Verification items for the finished model (mm, model axes). Coordinates: 2 decimals unless noted, no trailing zeros. Order: outer loops, then holes, each group sorted by start corner. A loop starts at its lowest first (then second) coordinate and runs counter-clockwise, first axis right, second up. Notation, with made-up numbers: M 32.5,32 L 56.5,32 A32 cw 56.5,66 Z; hole C 82,27 d5. An arc over 180 degrees is marked long. Use one line per item in the form item = value. Start each with the question number.
```python
from build123d import *

# Parameters (mm, degrees)
F0_W     = 15
F0_H     = 225
F1_DEPTH = 2


with BuildPart() as f1:
    # F0 (on Front) → F1 (new body)
    with BuildSketch(Plane.XZ):
        with Locations((7.5, 112.5)):
            Rectangle(F0_W, F0_H)
        with BuildLine():
            Line((4.5, 15), (4.5, 85))
            ThreePointArc((4.5, 85), (7.5, 88), (10.5, 85))
            Line((10.5, 85), (10.5, 15))
            ThreePointArc((10.5, 15), (7.5, 12), (4.5, 15))
        make_face(mode=Mode.SUBTRACT)
        with BuildLine():
            ThreePointArc((4.5, 210), (7.5, 213), (10.5, 210))
            Line((10.5, 210), (10.5, 140))
            ThreePointArc((10.5, 140), (7.5, 137), (4.5, 140))
            Line((4.5, 140), (4.5, 210))
        make_face(mode=Mode.SUBTRACT)
    extrude(amount=F1_DEPTH)


solid = f1.part
```
1. Material ranges on line 1 along X through (y, z) = (-1.2, 186); line 2 along Z through (x, y) = (7.75, -0.6); line 3 along Z through (x, y) = (9.25, -0.6), recorded low to high.
2. Cross-section at A-A on z = 82.5. Enter the section's corners in (x, y), and give its area (3 significant figures).
3. Cross-section at B-B on x = 7.5. Enter the section's corners in (y, z), and give its area (3 significant figures).
4. Cross-section at C-C on y = -1.65. Enter the section's corners in (x, z), and give its area (3 significant figures).
Final values:
q1.line_1 = 0 to 4.5, 10.5 to 15
q1.line_2 = 0 to 12.01, 87.99 to 137.01, 212.99 to 225
q1.line_3 = 0 to 12.56, 87.44 to 137.56, 212.44 to 225
q2.outline = M 0,-2 L 4.5,-2 L 4.5,0 L 0,0 Z; M 10.5,-2 L 15,-2 L 15,0 L 10.5,0 Z
q2.area = 18.0 mm2
q3.outline = M -2,0 L 0,0 L 0,12 L -2,12 Z; M -2,88 L 0,88 L 0,137 L -2,137 Z; M -2,213 L 0,213 L 0,225 L -2,225 Z
q3.area = 146 mm2
q4.outline = M 0,0 L 15,0 L 15,225 L 0,225 Z; hole M 4.5,15 A3 ccw 10.5,15 L 10.5,85 A3 ccw 4.5,85 Z; hole M 4.5,140 A3 ccw 10.5,140 L 10.5,210 A3 ccw 4.5,210 Z
q4.area = 2,480 mm2
